from build123d import *

# Parameters (mm, degrees)
F2_DEPTH  = 2
F3_W      = 8.4
F3_H      = 9.72
F4_DEPTH  = 2
F6_DEPTH  = 135.05
F7_DEPTH  = 19.271
F8_W      = 9.87
F8_H      = 34
F8_W_2    = 2
F9_DEPTH  = 1
F10_W     = 8.4
F10_H     = 1.15
F11_DEPTH = 2


with BuildPart() as f2:
    # F1 (on Top) → F2 (new body)
    with BuildSketch(Plane.XY):
        Polygon((-7.085, 9.87), (-68.3, 9.87), (-68.3, -24.13), (68.3, -24.13), (68.3, 9.87), (7.085, 9.87), (7.085, -7.13), (4.935, -7.13), (4.935, 9.87), (-4.935, 9.87), (-4.935, -7.13), (-7.085, -7.13), align=None)
    extrude(amount=F2_DEPTH)

    # F3 (on face) → F4 (join)
    with BuildSketch(Plane.XY.offset(2)):
        with Locations((-63.325, 0)):
            Rectangle(F3_W, F3_H)
        with Locations((-39.275, 0)):
            Rectangle(F3_W, F3_H)
        with Locations((39.275, 0)):
            Rectangle(F3_W, F3_H)
        with Locations((63.325, 0)):
            Rectangle(F3_W, F3_H)
    extrude(amount=F4_DEPTH)

    # F5 (on face) → F6 (join, through all)
    with BuildSketch(Plane(origin=(-67.525, 0, 0), x_dir=(0, -1, 0), z_dir=(-1, 0, 0))):
        Polygon((6.16, 4), (4.86, 4), (4.86, 3), align=None)
    extrude(amount=-F6_DEPTH)

    # F7 (cut, through all): faces of the model
    f7_faces = [f2.faces().sort_by_distance(p)[0] for p in [
        (-51.3, -4.86, 3.5),
        (0, -4.86, 3.5),
        (51.3, -4.86, 3.5),
    ]]
    extrude(f7_faces, amount=-F7_DEPTH, mode=Mode.SUBTRACT)

    # F8 (on face) → F9 (join)
    with BuildSketch(Plane.XY.offset(2)):
        with Locations((0, -7.13)):
            Rectangle(F8_W, F8_H)
        with Locations((-8.085, -7.13)):
            Rectangle(F8_W_2, F8_H)
        with Locations((8.085, -7.13)):
            Rectangle(F8_W_2, F8_H)
    extrude(amount=F9_DEPTH)

    # F10 (on face) → F11 (cut, through all)
    with BuildSketch(Plane.XY.offset(4)):
        with Locations((-63.325, 4.285)):
            Rectangle(F10_W, F10_H)
        with Locations((-39.275, 4.285)):
            Rectangle(F10_W, F10_H)
        with Locations((63.325, 4.285)):
            Rectangle(F10_W, F10_H)
        with Locations((39.275, 4.285)):
            Rectangle(F10_W, F10_H)
    extrude(amount=-F11_DEPTH, mode=Mode.SUBTRACT)


solid = f2.part
Source: CAD feature listing. Evaluate the final solid. Frame: model axes, mm. A direction names the side the tool comes from. Give positions to 0.01 mm unless a question says otherwise; leave off trailing zeros. Write each loop counter-clockwise with the first axis right and the second up, starting at its lowest first coordinate (ties: lowest second). Pieces come first, ordered by that corner, then holes. Notation, with made-up numbers: M 80.25,6.25 L 126.25,6.25 A15 ccw 126.25,30.25 Z; hole C -35.75,67 d1. An arc over 180 degrees is marked long. Return JSON: item names as keys, results as strings. Group by question number.
1) Ray query, L1, parallel to X at y = 7.5, z = 0.5 (3 decimals); L2, parallel to X at y = -12, z = 2.1 (3 decimals); L3, parallel to Z at x = -24.5, y = -14. Return the intervals inside material, ascending.
2) Cut plane A-A, the plane y = -3.5. Give the number of separate pieces and of enclosed holes in the cut face, then the cut area to 3 significant figures.
3) Draft query along X for faces 4 (the face through (0, -7, 3)), 5 (the face through (38, -7, 2)), 6 (the face through (63, -1, 4)). Return one class per face: released by +X, released by -X, zero draft, split by the parting line, or undercut.
4) Set-up query: faces 1 (the face through (6, -16, 2)), 2 (the face through (4.935, -4, 2)), 3 (the face through (-1, -24.13, 1)). Return all of +Z, -Z, +X, -X, +Y, -Y with unobstructed straight access to the full face (end or side cutting, diameter ignored); none if empty.
5) Cut plane D-D, the plane y = -11. Output: boundary loops of the cut face in (x, z) (3 decimals), then the cut area to 3 significant figures.
6) First-contact query: pin 1 Ø2.5 at (x, y) = (6, -16) entering from +Z; pin 2 Ø0.6 at (y, z) = (-2, 3.5) entering from -X (3 decimals); pin 3 Ø1.5 at (y, z) = (-10, 3.5) entering from -X (3 decimals). Flat tips, straight axial feed; report the tip coordinate or a pass-through.
7) Cut plane C-C, the plane x = 41. Output: boundary loops of the cut face in (y, z), then the cut area to 3 significant figures.
8) Cut plane B-B, the plane z = 1.15. Output: boundary loops of the cut face in (x, y) (3 decimals), then the cut area to 3 significant figures.
Data:
{
 "1": {"L1": "x = -68.3 to -7.085, -4.935 to 4.935, 7.085 to 68.3", "L2": "x = -9.085 to -7.085, -4.935 to 4.935, 7.085 to 9.085", "L3": "z = 0 to 2"},
 "2": {"separate pieces": "3", "enclosed holes": "0", "area": "346 mm²"},
 "3": {"face 4": "undercut", "face 5": "undercut", "face 6": "zero draft"},
 "4": {"face 1": "+Z, +Y, -Y", "face 2": "+Z, +Y", "face 3": "+Z, -Z, +X, -X, -Y"},
 "5": {"outline": "M -68.3,0 L 68.3,0 L 68.3,2 L 9.085,2 L 9.085,3 L 7.085,3 L 7.085,2 L 4.935,2 L 4.935,3 L -4.935,3 L -4.935,2 L -7.085,2 L -7.085,3 L -9.085,3 L -9.085,2 L -68.3,2 Z", "area": "287 mm²"},
 "6": {"pin 1": "stops at z = 3", "pin 2": "stops at x = -67.525", "pin 3": "stops at x = -9.085"},
 "7": {"outline": "M -24.13,0 L 9.87,0 L 9.87,2 L 3.71,2 L 3.71,4 L -6.16,4 L -4.86,3 L -4.86,2 L -24.13,2 Z", "area": "85.8 mm²"},
 "8": {"outline": "M -68.3,-24.13 L 68.3,-24.13 L 68.3,9.87 L 7.085,9.87 L 7.085,-7.13 L 4.935,-7.13 L 4.935,9.87 L -4.935,9.87 L -4.935,-7.13 L -7.085,-7.13 L -7.085,9.87 L -68.3,9.87 Z", "area": "4,570 mm²"}
}
